from build123d import *

# Parameters (mm, degrees)
SKETCH_1_W          = 31.8
SKETCH_1_H          = 31.8
EXTRUDE_1_DEPTH     = 3.2
SKETCH_2_W          = 16.2
SKETCH_2_H          = 16.2
CUT_EXTRUDE_3_DEPTH = 23.712551596
SKETCH_3_R          = 2.4
EXTRUDE_2_DEPTH     = 1.7
SKETCH_4_R          = 2.5
CUT_EXTRUDE_4_DEPTH = 1.8


with BuildPart() as part:
    # Эскиз1 → Бобышка-Вытянуть1 (new body)
    with BuildSketch(Plane(origin=(0, 0, 0), x_dir=(1, 0, 0), z_dir=(0, 1, 0))):
        Rectangle(SKETCH_1_W, SKETCH_1_H)
    extrude(amount=EXTRUDE_1_DEPTH)

    # Эскиз2 → Вырез-Вытянуть3 (cut, through all)
    with BuildSketch(Plane(origin=(0, 3.2, 0), x_dir=(1, 0, 0), z_dir=(0, 1, 0))):
        Rectangle(SKETCH_2_W, SKETCH_2_H)
    extrude(amount=-CUT_EXTRUDE_3_DEPTH, mode=Mode.SUBTRACT)

    # Эскиз3 → Бобышка-Вытянуть2 (add)
    with BuildSketch(Plane(origin=(0, 3.2, 0), x_dir=(1, 0, 0), z_dir=(0, 1, 0))):
        with Locations(Location((-12, 12, 0), (0, 0, 270))):
            Circle(SKETCH_3_R)
        with Locations(Location((-4.126, 12, 0), (0, 0, 270))):
            Circle(SKETCH_3_R)
        with Locations(Location((3.748, 12, 0), (0, 0, 270))):
            Circle(SKETCH_3_R)
        with Locations(Location((11.622, 12, 0), (0, 0, 270))):
            Circle(SKETCH_3_R)
        with Locations(Location((-12, 4.126, 0), (0, 0, 270))):
            Circle(SKETCH_3_R)
        with Locations(Location((-12, -3.748, 0), (0, 0, 270))):
            Circle(SKETCH_3_R)
        with Locations(Location((-12, -11.622, 0), (0, 0, 270))):
            Circle(SKETCH_3_R)
        with Locations(Location((-4.126, -11.622, 0), (0, 0, 270))):
            Circle(SKETCH_3_R)
        with Locations(Location((3.748, -11.622, 0), (0, 0, 270))):
            Circle(SKETCH_3_R)
        with Locations(Location((11.622, -11.622, 0), (0, 0, 270))):
            Circle(SKETCH_3_R)
        with Locations(Location((11.622, -3.748, 0), (0, 0, 270))):
            Circle(SKETCH_3_R)
        with Locations(Location((11.622, 4.126, 0), (0, 0, 270))):
            Circle(SKETCH_3_R)
    extrude(amount=EXTRUDE_2_DEPTH)

    # Эскиз4 → Вырез-Вытянуть4 (cut)
    with BuildSketch(Plane.XZ):
        with Locations(Location((-12, 12, 0), (0, 0, 270))):
            Circle(SKETCH_4_R)
        with Locations(Location((-4.126, 12, 0), (0, 0, 270))):
            Circle(SKETCH_4_R)
        with Locations(Location((3.748, 12, 0), (0, 0, 270))):
            Circle(SKETCH_4_R)
        with Locations(Location((11.622, 12, 0), (0, 0, 270))):
            Circle(SKETCH_4_R)
        with Locations(Location((-12, 4.126, 0), (0, 0, 270))):
            Circle(SKETCH_4_R)
        with Locations(Location((11.622, 4.126, 0), (0, 0, 270))):
            Circle(SKETCH_4_R)
        with Locations(Location((-12, -3.748, 0), (0, 0, 270))):
            Circle(SKETCH_4_R)
        with Locations(Location((11.622, -3.748, 0), (0, 0, 270))):
            Circle(SKETCH_4_R)
        with Locations(Location((-12, -11.622, 0), (0, 0, 270))):
            Circle(SKETCH_4_R)
        with Locations(Location((11.622, -11.622, 0), (0, 0, 270))):
            Circle(SKETCH_4_R)
        with Locations(Location((-4.126, -11.622, 0), (0, 0, 270))):
            Circle(SKETCH_4_R)
        with Locations(Location((3.748, -11.622, 0), (0, 0, 270))):
            Circle(SKETCH_4_R)
    extrude(amount=-CUT_EXTRUDE_4_DEPTH, mode=Mode.SUBTRACT)


solid = part.part
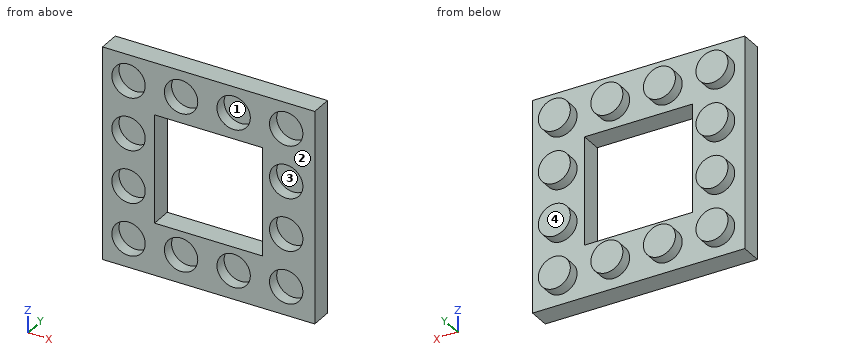
Check sheet for the modelled part. Datum: model origin and axes. Units: mm. Face numbers are marked on the shaded views. A direction names the side the tool comes from. Round coordinates to 2 decimals unless told otherwise and drop trailing zeros. Loops run counter-clockwise (first coordinate to the right, second up) from the corner with the lowest first, then second, coordinate; pieces in that order, holes last. Notation, with made-up numbers: M -7.75,23 L 46.25,23 A18 cw 46.25,32 Z; hole C -38.75,3 d7. An arc over 180 degrees is marked long. One line per item, written item: value.
(1) Sectioned sample at C-C, the plane y = 4.05. Count the separate pieces of the cut face and the enclosed holes in it, then the cut area to 3 significant figures.
Computed values:
separate pieces: 12
enclosed holes: 0
area: 217 mm^2
(2) Thickness scan on line 1 (Z direction, x = 7, y = 0.6); line 2 (X direction, y = 1.15, z = 12). Record the ranges inside material, lowest first.
Computed values:
line 1: z = -15.9 to -8.1, 8.1 to 15.9
line 2: x = -15.9 to -14.5, -9.5 to -6.63, -1.63 to 1.25, 6.25 to 9.12, 14.12 to 15.9
(3) Access from +Z, -Z, +X, -X, +Y, -Y to the whole of each face (thin tool, end or side, straight path). Record for the marked faces 1 and 2.
Computed values:
face 1: -Y
face 2: +Z, -Z, +X, -X, -Y
(4) Depth check by flat-ended pin: pin 1 Ø3 at (x, z) = (1, 7) entering from +Y; pin 2 Ø1.5 at (x, z) = (4.5, -10.5) entering from -Y. Enter the tip coordinate at first touch or a pass-through.
Computed values:
pin 1: stops at y = 3.2
pin 2: stops at y = 1.8
(5) Release check for a two-part mould opening along X. For the marked faces 3 and 4 record: +X half, -X half, draft (parallel to the pull), parting line (faces both ways), or undercut.
Computed values:
face 3: undercut
face 4: draft
(6) Sectioned sample at B-B, the plane z = 0. Record the cut outline in (x, y).
Computed values:
outline: M -15.9,0 L -8.1,0 L -8.1,3.2 L -15.9,3.2 Z; M 8.1,0 L 15.9,0 L 15.9,3.2 L 8.1,3.2 Z
(7) Sectioned sample at D-D, the plane x = -3.5. Record the cut outline in (y, z), then the cut area to 3 significant figures.
Computed values:
outline: M 0,-15.9 L 3.2,-15.9 L 3.2,-14.32 L 4.9,-14.32 L 4.9,-9.68 L 3.2,-9.68 L 3.2,-8.1 L 0,-8.1 L 0,-9.2 L 1.8,-9.2 L 1.8,-14.04 L 0,-14.04 Z; M 0,8.1 L 3.2,8.1 L 3.2,9.31 L 4.9,9.31 L 4.9,13.94 L 3.2,13.94 L 3.2,15.9 L 0,15.9 L 0,14.42 L 1.8,14.42 L 1.8,9.58 L 0,9.58 Z
area: 48.2 mm^2
(8) Sectioned sample at A-A, the plane x = 7.5. Record the cut outline in (y, z), then the cut area to 3 significant figures.
Computed values:
outline: M 0,-15.9 L 3.2,-15.9 L 3.2,-8.1 L 0,-8.1 Z; M 0,8.1 L 3.2,8.1 L 3.2,15.9 L 0,15.9 Z
area: 49.9 mm^2
